Can you work these out from the model? Positions are in its coordinate system, mm. Round coordinates to 2 decimals unless told otherwise and drop trailing zeros. Loops run counter-clockwise (first coordinate to the right, second up) from the corner with the lowest first, then second, coordinate; pieces in that order, holes last. Notation, with made-up numbers: (62, 15.25) -> (85, 15.25) arc R10 cw to (85, 20.25) -> close; hole circle Ø6 at (-21.75, 5). An arc over 180 degrees is marked (long way). Use a Markdown table: item, result.
from build123d import *

# Parameters (mm, degrees)
F1_DEPTH = 25.4


with BuildPart() as f1:
    # F0 (on Right) → F1 (new body)
    with BuildSketch(Plane.YZ):
        with BuildLine():
            Line((-10.786085, 37.710954), (-35.62377, 37.710954))
            Line((-35.62377, 37.710954), (-35.62377, 5.30417))
            Line((-35.62377, 5.30417), (-17.136085, 5.30417))
            ThreePointArc((-17.136085, 5.30417), (-12.645957, 7.164042), (-10.786085, 11.65417))
            Line((-10.786085, 11.65417), (-10.786085, 37.710954))
        make_face()
    extrude(amount=F1_DEPTH)


solid = f1.part
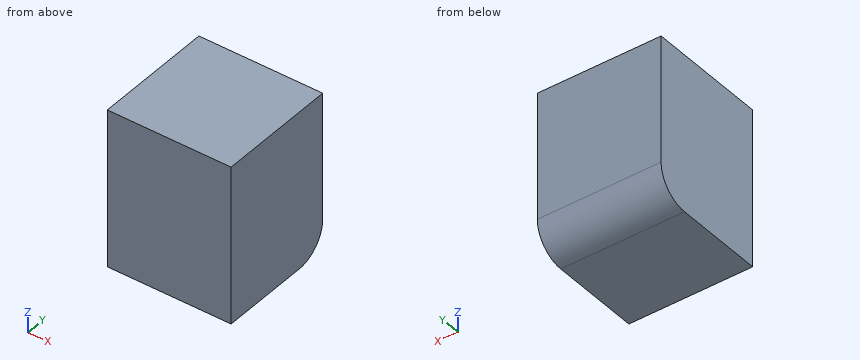
1. Will this pin go through, and if not, where does the flat tip stop? pin 1 Ø8 at (y, z) = (-14.5, 25) entering from -X.
Answer sheet:
| item | result |
|---|---|
| pin 1 | stops at x = 0 |
2. I need wall thicknesses on line 1 (Y direction, x = 1.25, z = 7); line 2 (Y direction, x = 20, z = 9.5); line 3 (Z direction, x = 11.75, y = -11.75). Which ranges of each line are inside material? Lowest first, please.
Answer sheet:
| item | result |
|---|---|
| line 1 | y = -35.62 to -12.82 |
| line 2 | y = -35.62 to -11.16 |
| line 3 | z = 8.29 to 37.71 |
3. I want a section at A-A (z = 8.5). Please give me the cut outline in (x, y), plus the area to 3 significant figures.
Answer sheet:
| item | result |
|---|---|
| outline | (0, -35.62) -> (25.4, -35.62) -> (25.4, -11.62) -> (0, -11.62) -> close |
| area | 610 mm² |
